from build123d import *

# Parameters (mm, degrees)
SKETCH1_R           = 6
BOSS_EXTRUDE1_DEPTH = 2.5
BOSS_EXTRUDE2_DEPTH = 7.5


with BuildPart() as part:
    # Sketch1 → Boss-Extrude1 (new, symmetric)
    with BuildSketch(Plane.XY):
        with BuildLine():
            Line((268.913125513, 20), (0, 20))
            ThreePointArc((0, 20), (-20, 0), (0, -20))
            Line((0, -20), (268.913125513, -20))
            ThreePointArc((268.913125513, -20), (279.827228639, -22.055727726), (289.245570139, -27.941176471))
            ThreePointArc((289.245570139, -27.941176471), (277, 0), (289.245570139, 27.941176471))
            ThreePointArc((289.245570139, 27.941176471), (279.827228639, 22.055727726), (268.913125513, 20))
        make_face()
        Circle(SKETCH1_R, mode=Mode.SUBTRACT)
    extrude(amount=BOSS_EXTRUDE1_DEPTH, both=True)

    # Sketch1_3 → Boss-Extrude2 (add, symmetric)
    with BuildSketch(Plane.XY):
        with BuildLine():
            ThreePointArc((289.245570139, 27.941176471), (280.195773714, 15.25338758), (277, 0))
            Line((277, 0), (319, 0))
            ThreePointArc((319, 0), (320.855462018, 9.451474044), (326.146428929, 17.5))
            Line((326.146428929, 17.5), (348.730549951, 17.5))
            ThreePointArc((348.730549951, 17.5), (321.56956349, 37.427808319), (289.245570139, 27.941176471))
        make_face()
        with BuildLine():
            Line((319, 0), (277, 0))
            ThreePointArc((277, 0), (280.195773714, -15.25338758), (289.245570139, -27.941176471))
            ThreePointArc((289.245570139, -27.941176471), (321.56956349, -37.427808319), (348.730549951, -17.5))
            Line((348.730549951, -17.5), (326.146428929, -17.5))
            ThreePointArc((326.146428929, -17.5), (320.855462018, -9.451474044), (319, 0))
        make_face()
    extrude(amount=BOSS_EXTRUDE2_DEPTH, both=True)


solid = part.part
Can you work these out from the model? Positions are in its coordinate system, mm. Give positions to 0.01 mm unless a question says otherwise; leave off trailing zeros. Order: outer loops, then holes, each group sorted by start corner. A loop starts at its lowest first (then second) coordinate and runs counter-clockwise, first axis right, second up. Notation, with made-up numbers: M 21,66.25 L 52,66.25 A14 ccw 52,78.25 Z; hole C -5.75,37.25 d6. An arc over 180 degrees is marked long. Use one line per item in the form item = value. Start each with the question number.
Item 1: We'd pull the mould along Y, two halves only. Please class faces 1 (the cylindrical face through (-20, 0, 0)), 2 (the flat face through (132, 0, 2.5)), 3 (the cylindrical face through (-6, 0, 0)): +Y half, -Y half, draft (parallel to the pull), parting line (faces both ways), or undercut.
Item 2: If I drill on line 1 along Y through (x, z) = (0, 1.55); line 2 along Z through (x, y) = (198.5, -16); line 3 along Y through (x, z) = (186.5, 1.25), over which ranges is the centre line in solid material (lowest first)?
Item 3: If we section it at A-A (z = -4.75): Write out the boundary of the cut face in (x, y).
Item 4: If we section it at B-B (x = 209.5): Write out the boundary of the cut face in (y, z).
Item 5: Will these pins go through, and if not, where does the flat tip stop? pin 1 Ø1 at (x, y) = (77.5, -4.5) entering from -Z; pin 2 Ø1.5 at (x, y) = (267, 5) entering from +Z; pin 3 Ø1 at (y, z) = (-24.5, 0.5) entering from +X.
Item 6: If we section it at C-C (y = -24): Write out the boundary of the cut face in (x, z).
Outcome:
q1.face_1 = parting line
q1.face_2 = draft
q1.face_3 = undercut
q2.line_1 = -20 to -6, 6 to 20
q2.line_2 = -2.5 to 2.5
q2.line_3 = -20 to 20
q3.outline = M 326.15,-17.5 A25 cw 326.15,17.5 L 348.73,17.5 A38 ccw long 348.73,-17.5 Z
q4.outline = M -20,-2.5 L 20,-2.5 L 20,2.5 L -20,2.5 Z
q5.pin_1 = -2.5
q5.pin_2 = 2.5
q5.pin_3 = 344.46
q6.outline = M 283.88,-2.5 L 285.54,-2.5 L 285.54,-7.5 L 344.46,-7.5 L 344.46,7.5 L 285.54,7.5 L 285.54,2.5 L 283.88,2.5 Z
